from build123d import *

# Parameters (mm, degrees)
F0_W      = 58.5
F0_H      = 91
F1_DEPTH  = 34
F2_T      = -1.5
F3_R      = 3
F4_R      = 2
F5_R      = 4
F6_DEPTH  = 34
F7_R      = 1.8
F8_DEPTH  = 32
F12_DEPTH = 4
F10_R     = 10.25
F13_DEPTH = 25


with BuildPart() as f1:
    # F0 (on Top) → F1 (new body)
    with BuildSketch(Plane.XY):
        Rectangle(F0_W, F0_H)
    extrude(amount=-F1_DEPTH)

    # F2
    f2_openings = [f1.faces().sort_by_distance(p)[0] for p in [
        (0, 0, 0),
    ]]
    offset(amount=F2_T, openings=f2_openings)

    # F3
    f3_edges = [f1.edges().sort_by_distance(p)[0] for p in [
        (-29.25, 45.5, -17),
        (29.25, 45.5, -17),
        (-29.25, -45.5, -17),
        (29.25, -45.5, -17),
    ]]
    fillet(f3_edges, radius=F3_R)

    # F4
    f4_edges = [f1.edges().sort_by_distance(p)[0] for p in [
        (-27.75, 44, -16.25),
        (-27.75, -44, -16.25),
        (27.75, -44, -16.25),
        (27.75, 44, -16.25),
    ]]
    fillet(f4_edges, radius=F4_R)

    # F5 (on face) → F6 (join)
    with BuildSketch(Plane.XY):
        with Locations((26.5, -42.5)):
            Circle(F5_R)
        with Locations((26.5, 42.5)):
            Circle(F5_R)
        with Locations((-26.5, 42.5)):
            Circle(F5_R)
        with Locations((-26.5, -42.5)):
            Circle(F5_R)
    extrude(amount=-F6_DEPTH)

    # F7 (on Top) → F8 (cut)
    with BuildSketch(Plane.XY):
        with Locations((26.5, -42.5)):
            Circle(F7_R)
        with Locations((26.5, 42.5)):
            Circle(F7_R)
        with Locations((-26.5, -42.5)):
            Circle(F7_R)
        with Locations((-26.5, 42.5)):
            Circle(F7_R)
    extrude(amount=-F8_DEPTH, mode=Mode.SUBTRACT)

    # F11 (on face) → F12 (join)
    with BuildSketch(Plane(origin=(0, 0, -34), x_dir=(1, 0, 0), z_dir=(0, 0, -1))):
        Polygon((26, -5), (29, -5), (29, 5), (26, 5), (26, 3), (27, 3), (27, -3), (26, -3), align=None)
        Polygon((1, 5), (1, -5), (4, -5), (4, -3), (3, -3), (3, 3), (4, 3), (4, 5), align=None)
    extrude(amount=-F12_DEPTH)

    # F10 (on face) → F13 (cut)
    with BuildSketch(Plane(origin=(0, 0, -34), x_dir=(1, 0, 0), z_dir=(0, 0, -1))):
        with Locations((15, 0)):
            Circle(F10_R)
    extrude(amount=-F13_DEPTH, mode=Mode.SUBTRACT)


solid = f1.part
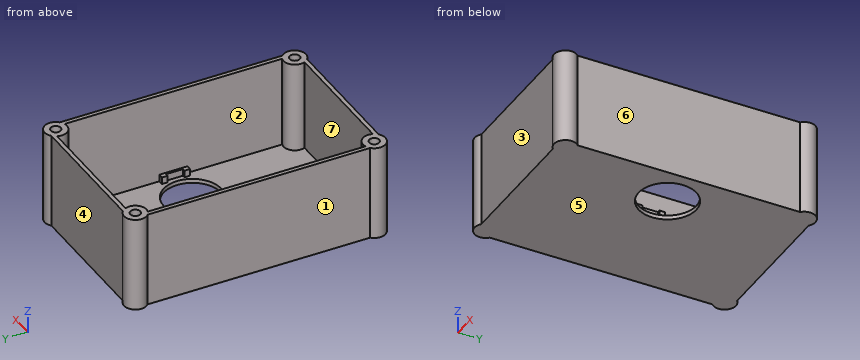
Part model, mm, in its own coordinate system. Face numbers are marked on the shaded views. A direction names the side the tool comes from. Coordinates: 2 decimals unless noted, no trailing zeros. Loops run counter-clockwise (first coordinate to the right, second up) from the corner with the lowest first, then second, coordinate; pieces in that order, holes last. Notation, with made-up numbers: M 54.5,-16.75 L 95.5,-16.75 A25 cw 95.5,1.25 Z; hole C -40,-3.75 d4. An arc over 180 degrees is marked long. Use a Markdown table: item, result. Add a question column.
Q1. Which spindle directions (+Z, -Z, +X, -X, +Y, -Y) get a long thin tool onto all of the face, cutting with end or side? Do the marked faces 1, 2, 3 and 4. Say none if no direction does.
Q2. Pin check, flat tips, straight feed: P1, Ø3, axis at y = 36.5, z = -10, coming from the +X side; P2, Ø2, axis at x = -26.5, y = 42.5, coming from the +Z side; P3, Ø4, axis at x = 18, z = -22, coming from the -Y side; P4, Ø1.8, axis at x = -25.5, y = 41.5, coming from the +Z side. Stop position of each tip, or through.
Q3. Probe L1, parallel to X at y = 38, z = -3; L2, parallel to Y at x = -10.5, z = -15; L3, parallel to Y at x = -25, z = -17. List the from-to ranges inside material, lowest first.
Q4. Cut at A-A (y = 0). Write the cut outline in (x, z), and give its area (3 significant figures).
Q5. Mould opens along X. For the marked faces 5, 6 and 7 say: +X half, -X half, draft (parallel to the pull), parting line (faces both ways), or undercut.
Q6. Cut at D-D (y = 42.5). Write the cut outline in (x, z), and give its area (3 significant figures).
Q7. Cut at C-C (z = -15.5). Write the cut outline in (x, y), and give its area (3 significant figures).
Q8. Cut at B-B (x = 15). Write the cut outline in (y, z), and give its area (3 significant figures).
Worked out:
| question | item | result |
|---|---|---|
| 1 | face 1 | +Z, -Z, -X |
| 1 | face 2 | +Z |
| 1 | face 3 | +Z, -Z, -Y |
| 1 | face 4 | +Z, -Z, +Y |
| 2 | P1 | stops at x = 29.25 |
| 2 | P2 | stops at z = -32 |
| 2 | P3 | stops at y = -45.5 |
| 2 | P4 | stops at z = 0 |
| 3 | L1 | x = -29.25 to -27.75, 27.75 to 29.25 |
| 3 | L2 | y = -45.5 to -44, 44 to 45.5 |
| 3 | L3 | y = -46.21 to -43.49, -41.51 to -38.79, 38.79 to 41.51, 43.49 to 46.21 |
| 4 | outline | M -29.25,-34 L 4.75,-34 L 4.75,-32.5 L 3,-32.5 L 3,-30 L 1,-30 L 1,-32.5 L -27.75,-32.5 L -27.75,0 L -29.25,0 Z; M 25.25,-34 L 29.25,-34 L 29.25,0 L 27.75,0 L 27.75,-30 L 27,-30 L 27,-32.5 L 25.25,-32.5 Z |
| 4 | area | 161 mm2 |
| 5 | face 5 | draft |
| 5 | face 6 | +X half |
| 5 | face 7 | undercut |
| 6 | outline | M -30.5,-34 L 30.5,-34 L 30.5,0 L 28.3,0 L 28.3,-32 L 24.7,-32 L 24.7,0 L 22.5,0 L 22.5,-32.5 L -22.5,-32.5 L -22.5,0 L -24.7,0 L -24.7,-32 L -28.3,-32 L -28.3,0 L -30.5,0 Z |
| 6 | area | 381 mm2 |
| 7 | outline | M -29.25,-39.6 A4 ccw -23.85,-45.5 L 23.85,-45.5 A4 ccw 29.25,-39.6 L 29.25,39.6 A4 ccw 23.85,45.5 L -23.85,45.5 A4 ccw -29.25,39.6 Z; hole C -26.5,-42.5 d3.6; hole C -26.5,42.5 d3.6; hole M -27.75,-38.7 A4 cw -22.79,-44 L 22.79,-44 A4 cw 27.75,-38.7 L 27.75,38.7 A4 cw 22.79,44 L -22.79,44 A4 cw -27.75,38.7 Z; hole C 26.5,-42.5 d3.6; hole C 26.5,42.5 d3.6 |
| 7 | area | 534 mm2 |
| 8 | outline | M -45.5,-34 L -10.25,-34 L -10.25,-32.5 L -44,-32.5 L -44,0 L -45.5,0 Z; M 10.25,-34 L 45.5,-34 L 45.5,0 L 44,0 L 44,-32.5 L 10.25,-32.5 Z |
| 8 | area | 203 mm2 |
